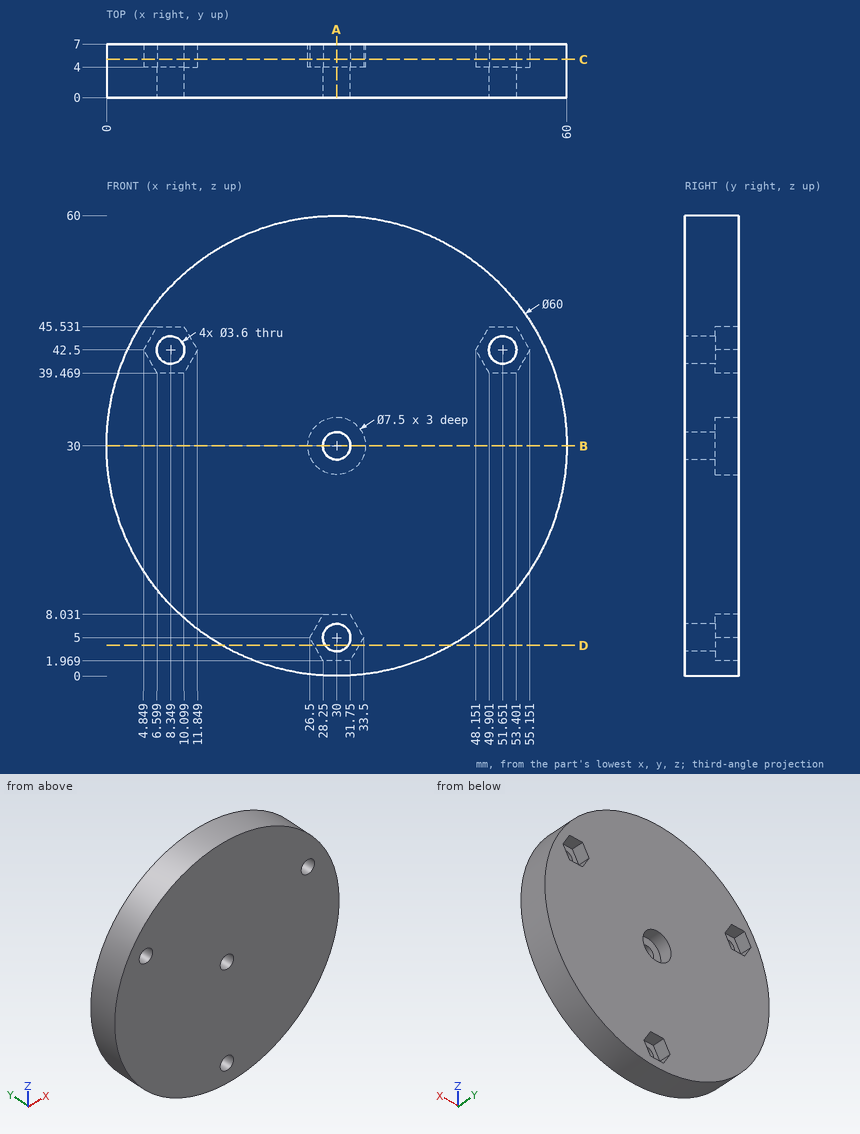
Could you check a few things on this drawing? It's one solid part, dimensions in mm from its lowest x, y, z. Round coordinates to 2 decimals unless told otherwise and drop trailing zeros. Loops run counter-clockwise (first coordinate to the right, second up) from the corner with the lowest first, then second, coordinate; pieces in that order, holes last. Notation, with made-up numbers: M 28.25,73.25 L 38.25,73.25 A23 cw 38.25,96.25 Z; hole C 43.25,11 d5. An arc over 180 degrees is marked long. Write item = value, one per line. Start each with the question number.
(1) I need wall thicknesses on line 1 along Z through (x, y) = (30, 6.4); line 2 along X through (y, z) = (1.75, 42.5); line 3 along Z through (x, y) = (51, 5.75) (1 decimal). Which ranges of each line are inside material? Lowest first, please.
(2) I'm going to push flat-ended pins straight in: P1, Ø2.5, axis at x = 51, y = 5.5, coming from the -Z side; P2, Ø2, axis at x = 16.5, y = 4, coming from the -Z side; P3, Ø0.9, axis at x = 30, y = 6, coming from the +Z side. Where does each tip first touch, or does it pass through?
(3) Suppose I cut it at C-C on y = 5. Write out the boundary of the cut face in (x, z).
(4) Suppose I cut it at D-D on z = 4. Write out the boundary of the cut face in (x, y).
(5) Suppose I cut it at A-A on x = 30. Write out the boundary of the cut face in (y, z).
(6) Suppose I cut it at B-B on z = 30. Write out the boundary of the cut face in (x, y).
Answer block:
q1.line_1 = 0 to 1.97, 8.03 to 26.25, 33.75 to 60
q1.line_2 = 2.73 to 6.55, 10.15 to 49.85, 53.45 to 57.27
q1.line_3 = 8.6 to 39.5, 45.5 to 51.4
q2.P1 = 7.42
q2.P2 = 2.73
q2.P3 = 60
q3.outline = C 30,30 d60; hole M 4.85,42.5 L 6.6,39.47 L 10.1,39.47 L 11.85,42.5 L 10.1,45.53 L 6.6,45.53 Z; hole C 30,30 d7.5; hole M 26.5,5 L 28.25,1.97 L 31.75,1.97 L 33.5,5 L 31.75,8.03 L 28.25,8.03 Z; hole M 48.15,42.5 L 49.9,39.47 L 53.4,39.47 L 55.15,42.5 L 53.4,45.53 L 49.9,45.53 Z
q4.outline = M 15.03,0 L 28.5,0 L 28.5,4 L 27.08,4 L 27.08,7 L 15.03,7 Z; M 31.5,0 L 44.97,0 L 44.97,7 L 32.92,7 L 32.92,4 L 31.5,4 Z
q5.outline = M 0,0 L 7,0 L 7,1.97 L 4,1.97 L 4,3.2 L 0,3.2 Z; M 0,6.8 L 4,6.8 L 4,8.03 L 7,8.03 L 7,26.25 L 4,26.25 L 4,28.2 L 0,28.2 Z; M 0,31.8 L 4,31.8 L 4,33.75 L 7,33.75 L 7,60 L 0,60 Z
q6.outline = M 0,0 L 28.2,0 L 28.2,4 L 26.25,4 L 26.25,7 L 0,7 Z; M 31.8,0 L 60,0 L 60,7 L 33.75,7 L 33.75,4 L 31.8,4 Z
